```python
from build123d import *

# Parameters (mm, degrees)
F1_DEPTH  = 25.4
F0_R      = 10.550798
F2_DEPTH  = 50.8
F4_DEPTH  = 6.35
F4_FACE_W = 6.35
F4_FACE_H = 20.509356
F5_DEPTH  = 2.54
F6_DEPTH  = 6.35


with BuildPart() as f1:
    # F0 (on Top) → F1 (new body)
    with BuildSketch(Plane.XY):
        with BuildLine():
            Line((-4.458389, 9.278268), (-59.164021, 9.278268))
            Line((-59.164021, 9.278268), (-59.164021, -12.170196))
            Line((-59.164021, -12.170196), (-4.458389, -12.170196))
            Line((-4.458389, -12.170196), (2.049189, -12.170196))
            ThreePointArc((2.049189, -12.170196), (-5.493572, -2.487583), (-1.999147, 9.278268))
            Line((-1.999147, 9.278268), (-4.458389, 9.278268))
        make_face()
    extrude(amount=F1_DEPTH)

    # F0 (on Top) → F2 (join)
    with BuildSketch(Plane.XY):
        with BuildLine():
            ThreePointArc((21.098027, 0), (12.685318, 12.445538), (-1.999147, 9.278268))
            ThreePointArc((-1.999147, 9.278268), (-5.493572, -2.487583), (2.049189, -12.170196))
            ThreePointArc((2.049189, -12.170196), (14.906878, -11.302344), (21.098027, 0))
        make_face()
        with Locations((7.685874, 0)):
            Circle(F0_R, mode=Mode.SUBTRACT)
    extrude(amount=F2_DEPTH)

    # F3 (on Front) → F4 (join)
    with BuildSketch(Plane.XZ):
        Polygon((-6.386341, 45.909356), (-43.499414, 24.460889), (-43.499414, 23.014925), (-6.386341, 23.014925), align=None)
    extrude(amount=F4_DEPTH)

    # F4_face (on face) → F5 (join)
    with BuildSketch(Plane(origin=(-6.386341, -3.175, 35.654678), x_dir=(0, 1, 0), z_dir=(1, 0, 0))):
        Rectangle(F4_FACE_W, F4_FACE_H)
    extrude(amount=F5_DEPTH)

    # F5_face (on face) → F6 (join)
    with BuildSketch(Plane(origin=(-17.779611, 0, 32.359046), x_dir=(1, 0, 0), z_dir=(0, 1, 0))):
        Polygon((11.39327, -13.55031), (12.053331, -13.55031), (12.053331, 6.959046), (-24.094825, 6.959046), align=None)
    extrude(amount=F6_DEPTH)


solid = f1.part
```
Input: part model. Units: mm. Frame: model coordinates. A direction names the side the tool comes from. Round coordinates to 2 decimals unless told otherwise and drop trailing zeros. Loops run counter-clockwise (first coordinate to the right, second up) from the corner with the lowest first, then second, coordinate; pieces in that order, holes last.
1) Pull-direction query (X, two-part tool) for faces 1 (the flat face through (-59.164, -1, 13)), 2 (the cylindrical face through (17.75, 3.17, 25.04)), 3 (the flat face through (-29, -12.17, 13)); classes: released by +X, released by -X, zero draft, split by the parting line, or undercut.
Ans:
face 1: released by -X
face 2: undercut
face 3: zero draft
2) Section query A-A on x = 3. Return the cut outline in (y, z), plus the area to 3 significant figures.
Ans:
outline: (-12.57, 0) - (-9.45, 0) - (-9.45, 50.8) - (-12.57, 50.8) - close; (9.45, 0) - (12.57, 0) - (12.57, 50.8) - (9.45, 50.8) - close
area: 316 mm2
3) Pin query (flat end, axial travel): pin 1 (6 mm diameter, centred on y = 6.5, z = 28, fed in from +X); pin 2 (4 mm diameter, centred on x = -46.5, y = -6.5, fed in from +Z); pin 3 (10 mm diameter, centred on x = -25, z = 38, fed in from +Y). Return the tip coordinate at first contact, or that it passes through.
Ans:
pin 1: stops at x = 20.63
pin 2: stops at z = 25.4
pin 3: stops at y = 6.35
4) Section query D-D on z = 41. Return the cut outline in (x, y).
Ans:
outline: (-14.88, -6.35) - (-4.13, -6.35) arc R13.41 ccw to (2.05, -12.17) arc R13.41 ccw (long way) to (-2, 9.28) arc R13.41 ccw to (-5.73, 0) - (-5.73, 6.35) - (-14.88, 6.35) - close; hole circle Ø21.1 at (7.69, 0)
5) Set-up query: faces 4 (the flat face through (-19, -6.35, 33)), 5 (the flat face through (-30, 9.278, 13)), 6 (the flat face through (14, -9, 50.8)), 7 (the flat face through (-29, 0, 0)), 8 (the flat face through (-20, 6.35, 33)). Return all of +Z, -Z, +X, -X, +Y, -Y with unobstructed straight access to the full face (end or side cutting, diameter ignored); none if empty.
Ans:
face 4: +Z, -X, -Y
face 5: +Z, -Z, -X, +Y
face 6: +Z, +X, -X, +Y, -Y
face 7: -Z, +X, -X, +Y, -Y
face 8: +Z, -X, +Y
6) Material intervals for line 1 (Y direction, x = -43, z = 23); line 2 (X direction, y = 8.25, z = 19); line 3 (Y direction, x = 7.5, z = 37), sorted ascending.
Ans:
line 1: y = -12.17 to 9.28
line 2: x = -59.16 to 1.11, 14.26 to 18.26
line 3: y = -13.41 to -10.55, 10.55 to 13.41
7) Section query B-B on z = 12.5. Return the cut outline in (x, y).
Ans:
outline: (-59.16, -12.17) - (2.05, -12.17) arc R13.41 ccw (long way) to (-2, 9.28) - (-59.16, 9.28) - close; hole circle Ø21.1 at (7.69, 0)
8) Section query C-C on x = -22.5. Return the cut outline in (y, z), plus the area to 3 significant figures.
Ans:
outline: (-12.17, 0) - (9.28, 0) - (9.28, 25.4) - (6.35, 25.4) - (6.35, 36.6) - (-6.35, 36.6) - (-6.35, 25.4) - (-12.17, 25.4) - close
area: 687 mm2
